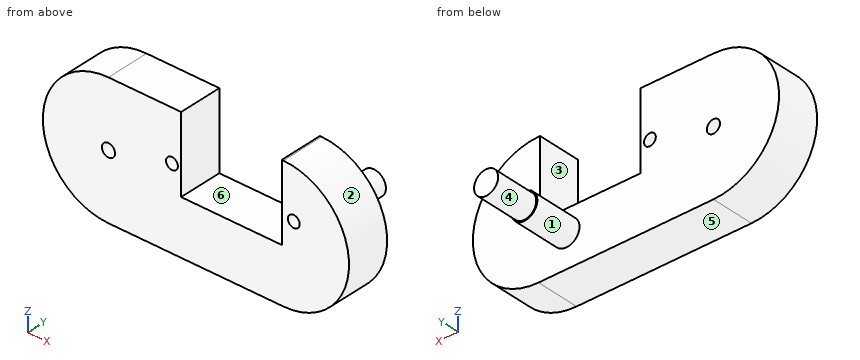
from build123d import *

# Parameters (mm, degrees)
SKETCH2_R            = 1.5
SKETCH2_R_2          = 1.35
BOSS_EXTRUDE5_DEPTH  = 10
SKETCH6_R            = 3
BOSS_EXTRUDE11_DEPTH = 24.05
SKETCH12_OUTSIDE_W   = 88.684
SKETCH12_OUTSIDE_H   = 48.684
SKETCH12_OUTSIDE_R   = 2.75
CUT_EXTRUDE10_DEPTH  = 13
SKETCH13_R           = 2.75
CUT_EXTRUDE11_DEPTH  = 3


with BuildPart() as part:
    # Sketch2 → Boss-Extrude5 (new body)
    with BuildSketch(Plane(origin=(0, 0, 0), x_dir=(1, 0, 0), z_dir=(0, 1, 0))):
        with BuildLine():
            Line((0, 15), (40, 15))
            ThreePointArc((40, 15), (55, 0), (40, -15))
            Line((40, -15), (39.620269747, -15))
            Line((39.620269747, -15), (39.620269747, -10))
            Line((39.620269747, -10), (39.620269747, 2.5))
            Line((39.620269747, 2.5), (16.620269747, 2.5))
            Line((16.620269747, 2.5), (16.620269747, -10))
            Line((16.620269747, -10), (16.620269747, -15))
            Line((16.620269747, -15), (0, -15))
            ThreePointArc((0, -15), (-15, 0), (0, 15))
        make_face()
        with Locations(Location((0, 0, 0), (0, 0, 270))):
            Circle(SKETCH2_R, mode=Mode.SUBTRACT)
        with Locations(Location((42.370269747, -3.5, 0), (0, 0, 270))):
            Circle(SKETCH2_R_2, mode=Mode.SUBTRACT)
        with Locations(Location((14.520269747, -3.5, 0), (0, 0, 270))):
            Circle(SKETCH2_R_2, mode=Mode.SUBTRACT)
    extrude(amount=BOSS_EXTRUDE5_DEPTH)

    # Sketch6 → Boss-Extrude11 (add)
    with BuildSketch(Plane(origin=(0, 10, 0), x_dir=(1, 0, 0), z_dir=(0, 1, 0))):
        with Locations(Location((33.620269747, 7.5, 0), (0, 0, 270))):
            Circle(SKETCH6_R)
    extrude(amount=BOSS_EXTRUDE11_DEPTH)

    # Sketch12 outside → Cut-Extrude10 (cut)
    with BuildSketch(Plane(origin=(0, 34.05, 0), x_dir=(1, 0, 0), z_dir=(0, 1, 0))):
        with Locations((20, 0)):
            Rectangle(SKETCH12_OUTSIDE_W, SKETCH12_OUTSIDE_H)
        with Locations(Location((33.620269747, 7.5, 0), (0, 0, 270))):
            Circle(SKETCH12_OUTSIDE_R, mode=Mode.SUBTRACT)
    extrude(amount=-CUT_EXTRUDE10_DEPTH, mode=Mode.SUBTRACT)

    # Sketch13 → Cut-Extrude11 (cut)
    with BuildSketch(Plane(origin=(0, 34.05, 0), x_dir=(1, 0, 0), z_dir=(0, 1, 0))):
        with Locations(Location((33.620269747, 7.5, 0), (0, 0, 270))):
            Circle(SKETCH13_R)
    extrude(amount=-CUT_EXTRUDE11_DEPTH, mode=Mode.SUBTRACT)


solid = part.part
Check sheet for the modelled part. Datum: model origin and axes. Units: mm. Face numbers are marked on the shaded views. A direction names the side the tool comes from. Round coordinates to 2 decimals unless told otherwise and drop trailing zeros. Order: outer loops, then holes, each group sorted by start corner. A loop starts at its lowest first (then second) coordinate and runs counter-clockwise, first axis right, second up. Notation, with made-up numbers: M 70,84.25 L 80,84.25 A25 ccw 80,114.25 Z; hole C 40.5,81.25 d1. An arc over 180 degrees is marked long. One line per item, written item: value. Start each with the question number.
1. Section check C-C on x = 21.5. Enter the section's corners in (y, z).
2. Release check for a two-part mould opening along X. For the marked faces 4, 5 and 6 record: released by +X, released by -X, zero draft, split by the parting line, or undercut.
3. Section check A-A on z = 0. Enter the section's corners in (x, y), and give its area (3 significant figures).
4. Gauge pin test, flat ends, axial feed: P1, Ø3, axis at x = 38, z = -11, coming from the +Y side; P2, Ø4, axis at x = 25, y = 8, coming from the +Z side; P3, Ø8, axis at x = 35, y = 24, coming from the -Z side; P4, Ø8, axis at x = 22, z = 1, coming from the -Y side. Record the tip position at first contact, or that the pin passes through.
5. Scan lines: line 1 along X through (y, z) = (4.5, 0); line 2 along X through (y, z) = (6, 3); line 3 along Y through (x, z) = (3, -11.5). Record each from-to range of solid material in increasing order.
6. Section check B-B on z = 12. Enter the section's corners in (x, y).
7. Section check D-D on z = 3.5. Enter the section's corners in (x, y), and give its area (3 significant figures).
8. Access from +Z, -Z, +X, -X, +Y, -Y to the whole of each face (thin tool, end or side, straight path). Record for the marked faces 1, 2 and 3.
Results found:
1. outline: M 0,-15 L 10,-15 L 10,-2.5 L 0,-2.5 Z
2. face 4: split by the parting line
2. face 5: zero draft
2. face 6: undercut
3. outline: M -15,0 L -1.5,0 L -1.5,10 L -15,10 Z; M 1.5,0 L 16.62,0 L 16.62,10 L 1.5,10 Z; M 39.62,0 L 55,0 L 55,10 L 39.62,10 Z
3. area: 440 mm^2
4. P1: y = 10
4. P2: z = -2.5
4. P3: z = -10.5
4. P4: y = 0
5. line 1: -15 to -1.5, 1.5 to 16.62, 39.62 to 55
5. line 2: -14.7 to 13.27, 15.77 to 16.62, 39.62 to 41.12, 43.62 to 54.7
5. line 3: 0 to 10
6. outline: M -9,0 L 16.62,0 L 16.62,10 L -9,10 Z; M 39.62,0 L 49,0 L 49,10 L 39.62,10 Z
7. outline: M -14.59,0 L 13.17,0 L 13.17,10 L -14.59,10 Z; M 15.87,0 L 16.62,0 L 16.62,10 L 15.87,10 Z; M 39.62,0 L 41.02,0 L 41.02,10 L 39.62,10 Z; M 43.72,0 L 54.59,0 L 54.59,10 L 43.72,10 Z
7. area: 408 mm^2
8. face 1: +Y
8. face 2: +X, +Y, -Y
8. face 3: +Z, +Y, -Y
